The figure shows three views and two pictorial views of one solid part (mm, origin at its lowest corner). Answer the questions. A direction names the side the tool comes from. Coordinates: 2 decimals unless noted, no trailing zeros. Loops run counter-clockwise (first coordinate to the right, second up) from the corner with the lowest first, then second, coordinate; pieces in that order, holes last. Notation, with made-up numbers: (-14.75, 23) -> (20.25, 23) arc R36 ccw to (20.25, 58) -> close; hole circle Ø1 at (56.25, 67.5). An arc over 180 degrees is marked (long way). Answer in a Markdown table with one row per item.
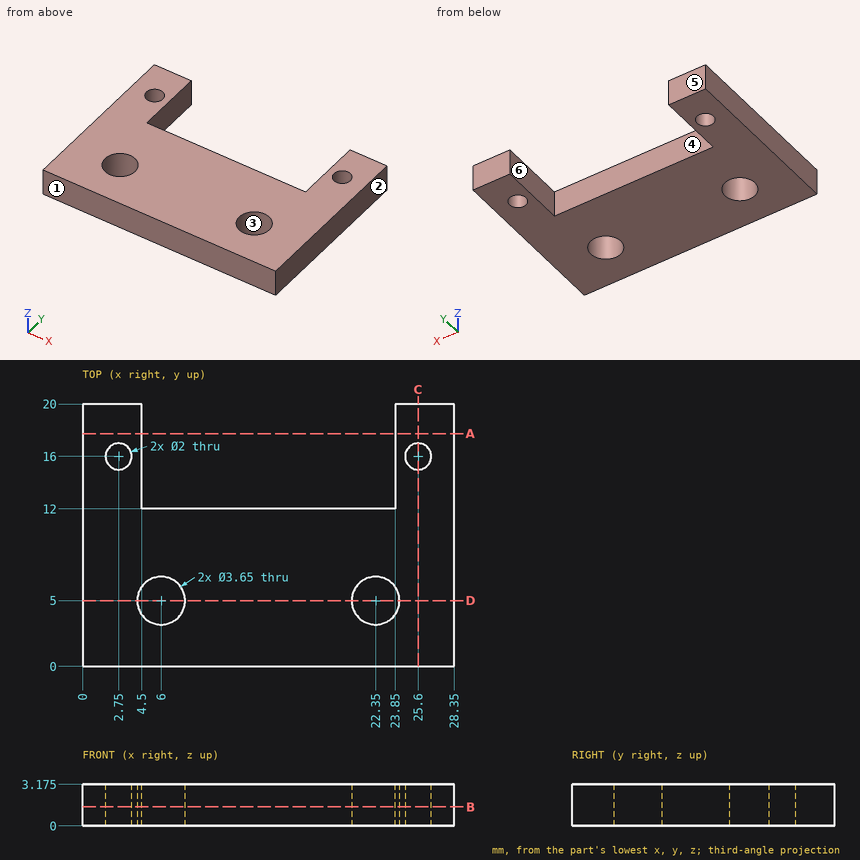
Item 1: Flat-ended cylindrical pins translate along their axes: pin 1 Ø10 at (x, y) = (8.5, 12.5) entering from -Z; pin 2 Ø2 at (x, y) = (6, 5) entering from -Z. Find the tip coordinate at first contact, or state that the pin passes through.
Findings below:
| item | result |
|---|---|
| pin 1 | stops at z = 0 |
| pin 2 | passes through |
Item 2: Find the intervals of material crossed by probe 1 along X at (y, z) = (17.75, 1.6); probe 2 along Y at (x, z) = (2.75, 0.8); probe 3 along Y at (x, z) = (6, 0.8) (3 decimals), in increasing order.
Findings below:
| item | result |
|---|---|
| probe 1 | x = 0 to 4.5, 23.85 to 28.35 |
| probe 2 | y = 0 to 15, 17 to 20 |
| probe 3 | y = 0 to 3.175, 6.825 to 12 |
Item 3: A cutting plane is placed at D-D, the plane y = 5. Determine the outline of the cut face in (x, z) (3 decimals), plus the area to 3 significant figures.
Findings below:
| item | result |
|---|---|
| outline | (0, 0) -> (4.175, 0) -> (4.175, 3.175) -> (0, 3.175) -> close; (7.825, 0) -> (20.525, 0) -> (20.525, 3.175) -> (7.825, 3.175) -> close; (24.175, 0) -> (28.35, 0) -> (28.35, 3.175) -> (24.175, 3.175) -> close |
| area | 66.8 mm2 |
Item 4: A tool of negligible diameter and unlimited length cuts with its end or side. For the marked faces 5 and 6, from which of +Z, -Z, +X, -X, +Y, -Y can it reach the whole face along a straight path? Write none if from no direction.
Findings below:
| item | result |
|---|---|
| face 5 | +Z, -Z, +X, -X, +Y |
| face 6 | +Z, -Z, +Y |
Item 5: Determine the mould class of the marked faces 1, 2, 3 and 4 for opening direction X: +X half, -X half, draft (parallel to the pull), parting line (faces both ways), or undercut.
Findings below:
| item | result |
|---|---|
| face 1 | draft |
| face 2 | +X half |
| face 3 | undercut |
| face 4 | undercut |
Item 6: A cutting plane is placed at B-B, the plane z = 1.45. Determine the outline of the cut face in (x, y) (3 decimals).
Findings below:
| item | result |
|---|---|
| outline | (0, 0) -> (28.35, 0) -> (28.35, 20) -> (23.85, 20) -> (23.85, 12) -> (4.5, 12) -> (4.5, 20) -> (0, 20) -> close; hole circle Ø2 at (2.75, 16); hole circle Ø3.65 at (6, 5); hole circle Ø3.65 at (22.35, 5); hole circle Ø2 at (25.6, 16) |
Item 7: A cutting plane is placed at C-C, the plane x = 25.6. Determine the outline of the cut face in (y, z) (3 decimals).
Findings below:
| item | result |
|---|---|
| outline | (0, 0) -> (15, 0) -> (15, 3.175) -> (0, 3.175) -> close; (17, 0) -> (20, 0) -> (20, 3.175) -> (17, 3.175) -> close |
Item 8: A cutting plane is placed at A-A, the plane y = 17.75. Determine the outline of the cut face in (x, z) (3 decimals).
Findings below:
| item | result |
|---|---|
| outline | (0, 0) -> (4.5, 0) -> (4.5, 3.175) -> (0, 3.175) -> close; (23.85, 0) -> (28.35, 0) -> (28.35, 3.175) -> (23.85, 3.175) -> close |
